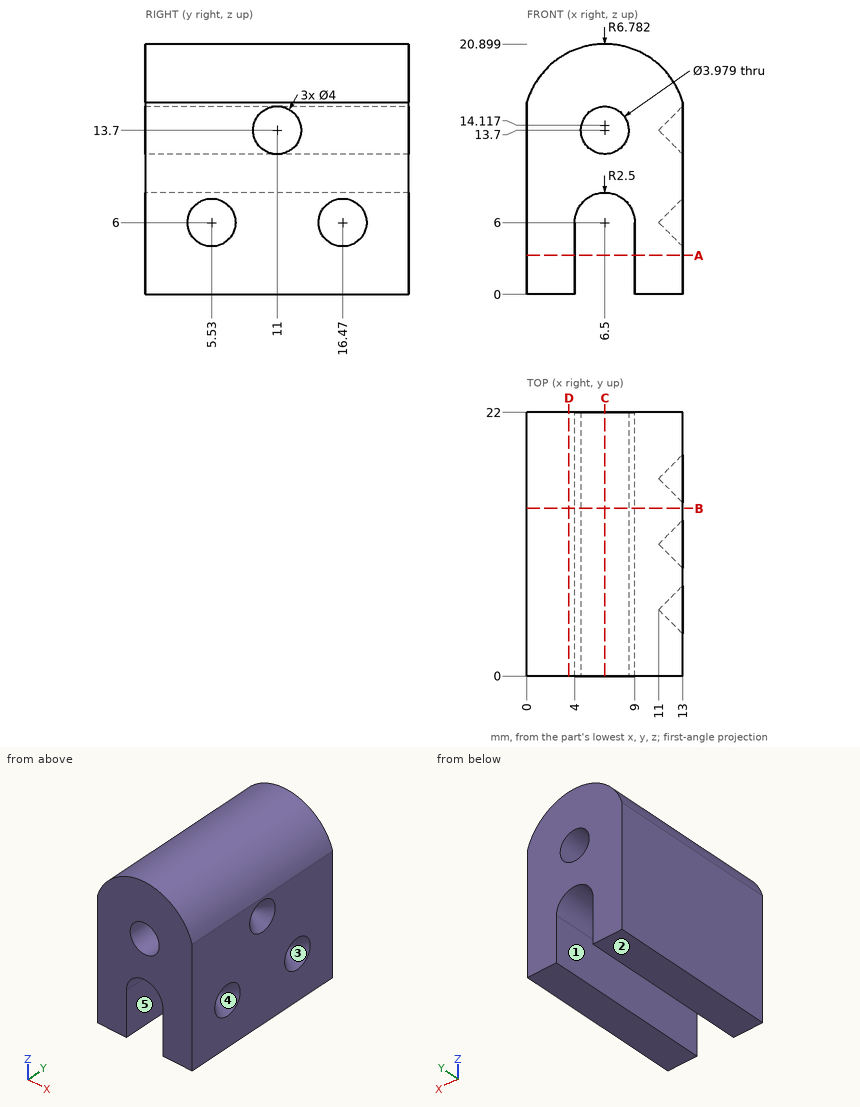
Check sheet for the drawn part. Datum: minimum x, y, z corner. Units: mm. A direction names the side the tool comes from. Give positions to 0.01 mm unless a question says otherwise; leave off trailing zeros. Order: outer loops, then holes, each group sorted by start corner. A loop starts at its lowest first (then second) coordinate and runs counter-clockwise, first axis right, second up. Notation, with made-up numbers: (-8, 76) - (12, 76) arc R9 ccw to (12, 86) - close; hole circle Ø4 at (-25, 69.25). An arc over 180 degrees is marked (long way). Write item = value, one per line. Start each with the question number.
1) Access from +Z, -Z, +X, -X, +Y, -Y to the whole of each face (thin tool, end or side, straight path). Record for the marked faces 4 and 5.
2) Draft check along X on the marked faces 1, 2 and 3. Enter one of: released by +X, released by -X, zero draft, split by the parting line, or undercut.
3) Section check C-C (x = 6.5). Enter the section's corners in (y, z).
4) Section check B-B (y = 14). Enter the section's corners in (x, z), then the cut area to 3 significant figures.
5) Section check A-A (z = 3.25). Enter the section's corners in (x, y).
6) Scan lines: L1, parallel to X at y = 21.25, z = 4.75; L2, parallel to X at y = 14.5, z = 13.7; L3, parallel to Z at x = 6.25, y = 16 (1 decimal). Record each from-to range of solid material in increasing order.
7) Section check D-D (x = 3.5). Enter the section's corners in (y, z), then the cut area to 3 significant figures.
8) Gauge pin test, flat ends, axial feed: pin 1 Ø1.5 at (y, z) = (19.5, 17) entering from -X; pin 2 Ø3 at (x, y) = (3.5, 14) entering from +Z. Record the tip position at first contact, or that the pin passes through.
Geometry check:
q1.face_4 = +X
q1.face_5 = -Z, +Y, -Y
q2.face_1 = undercut
q2.face_2 = zero draft
q2.face_3 = released by +X
q3.outline = (0, 8.5) - (22, 8.5) - (22, 11.71) - (0, 11.71) - close; (0, 15.69) - (22, 15.69) - (22, 20.9) - (0, 20.9) - close
q4.outline = (0, 0) - (4, 0) - (4, 6) arc R2.5 cw to (9, 6) - (9, 0) - (13, 0) - (13, 16.05) arc R6.78 ccw to (0, 16.05) - close; hole circle Ø3.98 at (6.5, 13.7)
q4.area = 203 mm2
q5.outline = (0, 0) - (4, 0) - (4, 22) - (0, 22) - close; (9, 0) - (13, 0) - (13, 22) - (9, 22) - close
q6.L1 = 0 to 4, 9 to 13
q6.L2 = 0 to 4.51, 8.49 to 13
q6.L3 = 8.5 to 11.7, 15.7 to 20.9
q7.outline = (0, 0) - (22, 0) - (22, 20.2) - (0, 20.2) - close
q7.area = 444 mm2
q8.pin_1 = 0.06
q8.pin_2 = 20.73
